Input: part model. Units: mm. Frame: model coordinates. A direction names the side the tool comes from. Round coordinates to 2 decimals unless told otherwise and drop trailing zeros. Loops run counter-clockwise (first coordinate to the right, second up) from the corner with the lowest first, then second, coordinate; pieces in that order, holes last. Notation, with made-up numbers: (-38.5, 12.25) -> (-9.5, 12.25) arc R27 cw to (-9.5, 45.25) -> close; hole circle Ø7 at (57, 42.25). An arc over 180 degrees is marked (long way). Answer as a JSON object with one key per item and string values. Group by question number.
Item 1: Draft query along Z for faces 1 (the flat face through (53, 0, 7)), 2 (the flat face through (43, -11.43, -33)), 3 (the flat face through (-38, -6, 38)). Return one class per face: released by +Z, released by -Z, zero draft, split by the parting line, or undercut.
Item 2: Section query C-C on y = -5.75. Count the separate pieces of the cut face and the enclosed holes in it, and give its area (3 significant figures).
Item 3: Material intervals for line 1 (Z direction, x = -1, y = -6.25); line 2 (Z direction, x = -45.5, y = 3); line 3 (Y direction, x = 39, z = -41.5), sorted ascending. Write a range as [from, to].
Item 4: Section query A-A on x = -17.5. Return loops of the section in (y, z), and give its area (3 significant figures).
Item 5: Section query D-D on x = -46. Return loops of the section in (y, z), and give its area (3 significant figures).
Item 6: Section query B-B on z = 22.5. Return loops of the section in (x, y), and give its area (3 significant figures).
Item 7: Set-up query: faces 4 (the flat face through (-33, 0, 43)), 5 (the flat face through (-38, -6, -38)), 6 (the flat face through (38, -6, 38)). Return all of +Z, -Z, +X, -X, +Y, -Y with unobstructed straight access to the full face (end or side cutting, diameter ignored); none if empty.
Item 8: Pin query (flat end, axial travel): pin 1 (5 mm diameter, centred on x = 52.5, y = -7.5, fed in from +Z); pin 2 (3 mm diameter, centred on y = -3.5, z = -20, fed in from -X); pin 3 (3 mm diameter, centred on x = 27.5, y = 0, fed in from -Z). Return the tip coordinate at first contact, or that it passes through.
Autodesk Inventor part; units mm, degrees
ref_plane "YZ Plane" through (0, 0, 0) normal (1, 0, 0) x (0, 1, 0)
ref_plane "XZ Plane" through (0, 0, 0) normal (0, 1, 0) x (-1, 0, 0)
ref_plane "XY Plane" through (0, 0, 0) normal (0, 0, 1) x (1, 0, 0)
sketch "Sketch1" plane through (0, 0, 0) normal (0, 1, 0) x (-1, 0, 0)
  circle A0 centre (0, 0) radius 57.15
  circle A1 centre (0, 0) radius 50.8
  line L0 (0, 0) -> (0, -57.15)
  line L1 (0, 0) -> (57.15, 0) construction
  line L2 (49.069, -13.148) -> (55.2027, -14.7915)
  line L3 (0, 0) -> (57.15, 0) construction
  line L4 (0, 0) -> (57.15, 0)
  line L5 (43.9941, -25.4) -> (49.4934, -28.575)
  line L6 (0, 0) -> (57.15, 0) construction
  line L7 (50.8, 0) -> (57.15, 0)
  line L8 (49.069, 13.148) -> (55.2027, 14.7915)
  line L9 (43.9941, 25.4) -> (49.4934, 28.575)
  line L10 (35.921, 35.921) -> (40.4112, 40.4112)
  line L11 (25.4, 43.9941) -> (28.575, 49.4934)
  line L12 (13.148, 49.069) -> (14.7915, 55.2027)
  line L13 (0, 50.8) -> (0, 57.15)
  line L14 (-13.148, 49.069) -> (-14.7915, 55.2027)
  line L15 (-25.4, 43.9941) -> (-28.575, 49.4934)
  line L16 (-35.921, 35.921) -> (-40.4112, 40.4112)
  line L17 (-43.9941, 25.4) -> (-49.4934, 28.575)
  line L18 (-49.069, 13.148) -> (-55.2027, 14.7915)
  line L19 (-50.8, 0) -> (-57.15, 0)
  line L20 (-49.069, -13.148) -> (-55.2027, -14.7915)
  line L21 (-43.9941, -25.4) -> (-49.4934, -28.575)
  line L22 (-35.921, -35.921) -> (-40.4112, -40.4112)
  line L23 (-25.4, -43.9941) -> (-28.575, -49.4934)
  line L24 (-13.148, -49.069) -> (-14.7915, -55.2027)
  line L25 (0, -50.8) -> (0, -57.15)
  line L26 (13.148, -49.069) -> (14.7915, -55.2027)
  line L27 (25.4, -43.9941) -> (28.575, -49.4934)
  line L28 (35.921, -35.921) -> (40.4112, -40.4112)
  point P0 (50.8, 0)
  point P1 (0, -50.8)
  dimension "d0" = 114.3
  dimension "d1" = 101.6
  dimension "d3" = 15
  dimension "d4" = 30
  dimension "d7" = 360
extrude "Extrusion1" add sketch "Sketch1" along normal blind 6.35 contours L4 A1 L8 A0 | A0 L2 A1 L4 | L8 A1 L9 A0 | A0 L5 A1 L2 | L9 A1 L10 A0 | A0 L28 A1 L5 | L10 A1 L11 A0 | A0 L27 A1 L28 | L0 A0 L24 A1 | A1 L26 A0 L0 | L11 A1 L12 A0 | A0 L26 A1 L27 | L24 A0 L23 A1 | L12 A1 L13 A0 | L23 A0 L22 A1 | L13 A1 L14 A0 | L22 A0 L21 A1 | L14 A1 L15 A0 | L21 A0 L20 A1 | L15 A1 L16 A0 | L20 A0 L19 A1 | L16 A1 L17 A0 | L19 A0 L18 A1 | L17 A1 L18 A0
extrude "Extrusion2" add sketch "Sketch1" against normal blind 11.43 contours L4 A1 L8 A0 | A0 L5 A1 L2 | L9 A1 L10 A0 | A0 L27 A1 L28 | A1 L26 A0 L0 | L11 A1 L12 A0 | L24 A0 L23 A1 | L13 A1 L14 A0 | L22 A0 L21 A1 | L15 A1 L16 A0 | L20 A0 L19 A1 | L17 A1 L18 A0
properties part number "4 Castle Spacer"
Solved:
{
 "1": {"face 1": "undercut", "face 2": "zero draft", "face 3": "released by +Z"},
 "2": {"separate pieces": "12", "enclosed holes": "0", "area": "1,080 mm²"},
 "3": {"line 1": "[-57.14, -50.79]", "line 2": "[-34.58, -22.59], [22.59, 34.58]", "line 3": "[0, 6.35]"},
 "4": {"outline": "(-11.43, 47.69) -> (6.35, 47.69) -> (6.35, 54.4) -> (-11.43, 54.4) -> close; (0, -54.4) -> (6.35, -54.4) -> (6.35, -47.69) -> (0, -47.69) -> close", "area": "162 mm²"},
 "5": {"outline": "(-11.43, -26.56) -> (0, -26.56) -> (0, -33.91) -> (6.35, -33.91) -> (6.35, -21.56) -> (-11.43, -21.56) -> close; (-11.43, 26.56) -> (0, 26.56) -> (0, 21.56) -> (6.35, 21.56) -> (6.35, 33.91) -> (-11.43, 33.91) -> close", "area": "298 mm²"},
 "6": {"outline": "(-52.53, 0) -> (-45.55, 0) -> (-45.55, 6.35) -> (-52.53, 6.35) -> close; (45.55, -11.43) -> (52.53, -11.43) -> (52.53, 6.35) -> (45.55, 6.35) -> close", "area": "169 mm²"},
 "7": {"face 4": "-Y", "face 5": "-X, -Y", "face 6": "+X, -Y"},
 "8": {"pin 1": "z = 27.68", "pin 2": "x = -54.07", "pin 3": "z = -50.89"}
}
